CAD build for the part. Positions are in the model's coordinates, mm. A direction names the side the tool comes from. Coordinates: 2 decimals unless noted, no trailing zeros. Loops run counter-clockwise (first coordinate to the right, second up) from the corner with the lowest first, then second, coordinate; pieces in that order, holes last. Notation, with made-up numbers: (40.25, 54.5) -> (59.25, 54.5) arc R14 cw to (59.25, 63.5) -> close; hole circle Ø10 at (89, 0). An arc over 180 degrees is marked (long way). Write item = value, one per line. Start each with the question number.
(1) Band-saw the part on A-A (y = -5). Write the cut outline in (x, z).
(2) Drill centre lines: line 1 (Z direction, x = -132.75, y = -5); line 2 (X direction, y = -6, z = 8); line 3 (Y direction, x = -44, z = 9.5). Where is each one in solid material? Low to high. Write a range as from..to.
(3) Band-saw the part on C-C (x = -54). Write the cut outline in (y, z).
(4) Tool access for faces 4 (the face through (-71, 10, 5)), 5 (the face through (-130, -2.7, 2.7)), 6 (the face through (0, 8.4, 2.7)): list every direction of +Z, -Z, +X, -X, +Y, -Y with a clear straight run to the whole face (end or side of a thin tool).
(5) Pull direction Z, two halves, no side cores. Call faces 1 (the face through (20, 5, 5)), 2 (the face through (-134.93, -3.616, 2.338)), 3 (the face through (-69, 5, 10)): +Z half, -Z half, draft (parallel to the pull), parting line (faces both ways), or undercut.
(6) Flat gauge pin, fed straight in: P1, Ø1.5, axis at y = -6, z = 2.5, coming from the +X side. Where does the tip first touch, or does it go through?
(7) Band-saw the part on B-B (z = 5). Write the cut outline in (x, y).
(8) Band-saw the part on D-D (y = 5). Write the cut outline in (x, z), and give its area (3 significant figures).
```python
from build123d import *

# Parameters (mm, degrees)
BOSS_EXTRUDE1_DEPTH = 10
SKETCH4_R           = 3
CUT_EXTRUDE2_DEPTH  = 150
SKETCH4_5_R         = 3
BOSS_EXTRUDE3_DEPTH = 20
CUT_EXTRUDE4_START  = -2
SKETCH5_R           = 3.5
SKETCH5_R_2         = 3
CUT_EXTRUDE4_DEPTH  = 2
FILLET2_R           = 12


with BuildPart() as part:
    # Sketch1 → Boss-Extrude1 (new body)
    with BuildSketch(Plane.XY):
        Polygon((-140, 10), (0, 10), (0, 0), (-130, 0), (-130, -10), (-140, -10), align=None)
    extrude(amount=BOSS_EXTRUDE1_DEPTH)

    # Sketch4 → Cut-Extrude2 (cut)
    with BuildSketch(Plane(origin=(0, 0, 0), x_dir=(0, 0, -1), z_dir=(1, 0, 0))):
        with Locations(Location((-5, -5, 0), (0, 0, 90))):
            Circle(SKETCH4_R)
    extrude(amount=-CUT_EXTRUDE2_DEPTH, mode=Mode.SUBTRACT)

    # Sketch4<5> → Boss-Extrude3 (add)
    with BuildSketch(Plane(origin=(0, 0, 0), x_dir=(0, 0, -1), z_dir=(1, 0, 0))):
        with Locations((-5, 5)):
            Circle(SKETCH4_5_R)
    extrude(amount=BOSS_EXTRUDE3_DEPTH)

    # Sketch5 → Cut-Extrude4 (cut)
    with BuildSketch(Plane(origin=(0, 0, 0), x_dir=(0, 0, -1), z_dir=(1, 0, 0)).offset(CUT_EXTRUDE4_START)):
        with Locations(Location((-5, 5, 0), (0, 0, 90))):
            Circle(SKETCH5_R)
        with Locations(Location((-5, 5, 0), (0, 0, 90))):
            Circle(SKETCH5_R_2, mode=Mode.SUBTRACT)
    extrude(amount=CUT_EXTRUDE4_DEPTH, mode=Mode.SUBTRACT)

    # Fillet2
    # the kernel refuses this fillet: 12 mm, written as the material it adds along each edge
    with BuildSketch(Plane(origin=(-2, 5, 5), x_dir=(0, 1, 0), z_dir=(0, 0, -1))) as fillet2_piece_1:
        with BuildLine():
            CenterArc((15, 3.4278273), FILLET2_R, 180, 16.597842136)
            Line((3, 3.4278273), (2.76, 3.4278273))
            Line((2.76, 3.4278273), (2.76, 0))
            Line((2.76, 0), (3, -0.24))
            ThreePointArc((3, -0.24), (3.25, -0.24), (3.27, -0.068556546))
            Line((3.27, -0.068556546), (3.5, 0))
        make_face()
    revolve(axis=Axis((-2, 5, 5), (1, 0, 0)))


solid = part.part
```
Findings below:
q1.outline = (-140, 0) -> (-130, 0) -> (-130, 2) -> (-140, 2) -> close; (-140, 8) -> (-130, 8) -> (-130, 10) -> (-140, 10) -> close
q2.line_1 = 0..2, 8..10
q2.line_2 = -140..-130
q2.line_3 = 0..10
q3.outline = (0, 0) -> (10, 0) -> (10, 10) -> (0, 10) -> close
q4.face_4 = +Z, -Z, +X, -X, +Y
q4.face_5 = +Z, -Z, +X, -Y
q4.face_6 = +X
q5.face_1 = draft
q5.face_2 = undercut
q5.face_3 = +Z half
q6.P1 = -130
q7.outline = (-140, -10) -> (-130, -10) -> (-130, -8) -> (-140, -8) -> close; (-140, -2) -> (-130, -2) -> (-130, 0) -> (0, 0) -> (0, 1.5) -> (-2, 1.5) arc R12 cw to (1.43, 2) -> (20, 2) -> (20, 8) -> (1.43, 8) arc R12 cw to (-2, 8.5) -> (0, 8.5) -> (0, 10) -> (-140, 10) -> close
q8.outline = (-140, 0) -> (0, 0) -> (0, 1.5) -> (-2, 1.5) arc R12 cw to (1.43, 2) -> (20, 2) -> (20, 8) -> (1.43, 8) arc R12 cw to (-2, 8.5) -> (0, 8.5) -> (0, 10) -> (-140, 10) -> close
q8.area = 1,520 mm²
